For this review, take the finished solid that the model builds, in its own axes (mm). A direction names the side the tool comes from. Coordinates: 2 decimals unless noted, no trailing zeros. Order: outer loops, then holes, each group sorted by start corner. A loop starts at its lowest first (then second) coordinate and runs counter-clockwise, first axis right, second up. Notation, with made-up numbers: (-5, -20.75) -> (1, -20.75) arc R9 ccw to (1, -13.75) -> close; hole circle Ø4 at (69.25, 39.5). An arc over 180 degrees is marked (long way). Return JSON: item names as keys, results as strings. Group by question number.
Item 1: Take a section at A-A (z = 3.5). Write out the cut boundary in (x, y) (3 decimals).
Item 2: Take a section at B-B (y = 28). Write out the cut boundary in (x, z) (3 decimals), then the cut area to 3 significant figures.
Item 3: Take a section at D-D (z = 66). Write out the cut boundary in (x, y) (3 decimals), then the cut area to 3 significant figures.
Item 4: For line 1 along Z through (x, y) = (-18, -22) (3 decimals); line 2 along Y through (x, z) = (35, 49.5); line 3 along Y through (x, z) = (-22, 13.5), list the stretches that pass through material, from the lowest coordinate up.
Item 5: Insertion check: pin 1 (16.5 mm diameter, centred on x = 12, y = 40.5, fed in from +Z) (3 decimals); pin 2 (15.5 mm diameter, centred on x = 43.5, z = 38, fed in from +Y); pin 3 (12 mm diameter, centred on x = 97, y = 10.5, fed in from -Z). Each pin has a flat end and moves straight along its axis. Give the tip position at first contact, or say it passes through.
Item 6: Machinability: for faces 1 (the flat face through (72, 0, 42.875)), 2 (the flat face through (-4, 7.938, 30)), 3 (the flat face through (62, 0, 61.925)), which of the approach directions +Z, -Z, +X, -X, +Y, -Y give a long, thin tool a straight path to every point of the face, cutting with its end or side? Answer none if there is none.
Item 7: Take a section at C-C (x = 101). Write out the cut boundary in (y, z).
```python
from build123d import *

# Parameters (mm, degrees)
F1_DEPTH = 63.5
F0_W     = 26.5017113779
F0_H     = 17.3551412069
F2_DEPTH = 25.4
F3_DEPTH = 7.9375
F5_R     = 6.35


with BuildPart() as f1:
    # F0 (on Front) → F1 (new body, symmetric)
    with BuildSketch(Plane.XZ):
        Polygon((-41.275, -9.525), (41.275, -9.525), (41.275, 9.525), (22.225, 9.525), (-41.275, 9.525), align=None)
    extrude(amount=F1_DEPTH, both=True)

    # F0 (on Front) → F2 (join, symmetric)
    with BuildSketch(Plane.XZ):
        with BuildLine():
            Line((22.225, 9.525), (41.275, 9.525))
            Line((41.275, 9.525), (41.275, 27.0002))
            ThreePointArc((41.275, 27.0002), (45.9246798487, 38.2255201513), (57.15, 42.8752))
            Line((57.15, 42.8752), (86.8267113779, 42.8752))
            Line((86.8267113779, 42.8752), (86.8267113779, 44.5700587931))
            Line((86.8267113779, 44.5700587931), (60.325, 44.5700587931))
            Line((60.325, 44.5700587931), (60.325, 61.9252))
            Line((60.325, 61.9252), (57.15, 61.9252))
            add(Edge.make_bspline(
                [(52.6432559299, 61.6332027992), (54.1237485825, 61.7442374051), (55.6258441188, 61.8416233146), (57.15, 61.9252)],
                knots=[108.3100725279, 108.3100725279, 108.3100725279, 108.3100725279, 111.5045361635, 111.5045361635, 111.5045361635, 111.5045361635], degree=3))
            ThreePointArc((52.6432559299, 61.6332027992), (30.9092524721, 50.0475164203), (22.225, 27.0002))
            Line((22.225, 27.0002), (22.225, 9.525))
        make_face()
        with Locations((73.5758556889, 53.2476293965)):
            Rectangle(F0_W, F0_H)
    extrude(amount=F2_DEPTH, both=True)

    # F0 (on Front) → F3 (join, symmetric)
    with BuildSketch(Plane.XZ):
        with BuildLine():
            add(Edge.make_bspline(
                [(-41.275, 9.525), (-22.9162119867, 38.413460075), (2.4463262192, 57.8685125131), (52.6432559299, 61.6332027992)],
                knots=[0, 0, 0, 0, 108.3100725279, 108.3100725279, 108.3100725279, 108.3100725279], degree=3))
            Line((-41.275, 9.525), (22.225, 9.525))
            Line((22.225, 9.525), (22.225, 27.0002))
            ThreePointArc((22.225, 27.0002), (30.9092524721, 50.0475164203), (52.6432559299, 61.6332027992))
        make_face()
    extrude(amount=F3_DEPTH, both=True)

    # F0 (on Front) → F4 (revolve)
    with BuildSketch(Plane.XZ):
        Polygon((86.8267113779, 61.9252), (86.8267113779, 44.5700587931), (111.125, 44.5700587931), (111.125, 73.1450587931), (86.8267113779, 73.1450587931), align=None)
    revolve(axis=Axis((86.8267113779, 0, 58.0101293965), (0, 0, 1)))

    # F5
    f5_edges = [f1.edges().sort_by_distance(p)[0] for p in [
        (41.275, -63.5, 0),
        (-41.275, -63.5, 0),
        (41.275, 63.5, 0),
        (-41.275, 63.5, 0),
    ]]
    fillet(f5_edges, radius=F5_R)


solid = f1.part
```
Findings below:
{
 "1": {"outline": "(-41.275, -57.15) arc R6.35 ccw to (-34.925, -63.5) -> (34.925, -63.5) arc R6.35 ccw to (41.275, -57.15) -> (41.275, 57.15) arc R6.35 ccw to (34.925, 63.5) -> (-34.925, 63.5) arc R6.35 ccw to (-41.275, 57.15) -> close"},
 "2": {"outline": "(-41.275, -9.525) -> (41.275, -9.525) -> (41.275, 9.525) -> (-41.275, 9.525) -> close", "area": "1,570 mm2"},
 "3": {"outline": "circle Ø48.597 at (86.827, 0)", "area": "1,850 mm2"},
 "4": {"line 1": "z = -9.525 to 9.525", "line 2": "y = -25.4 to 25.4", "line 3": "y = -7.94 to 7.94"},
 "5": {"pin 1": "stops at z = 9.525", "pin 2": "stops at y = 25.4", "pin 3": "stops at z = 44.57"},
 "6": {"face 1": "-Z, +X, +Y, -Y", "face 2": "+Z, -X, +Y", "face 3": "+Z, -X"},
 "7": {"outline": "(-19.74, 44.57) -> (19.74, 44.57) -> (19.74, 73.15) -> (-19.74, 73.15) -> close"}
}
